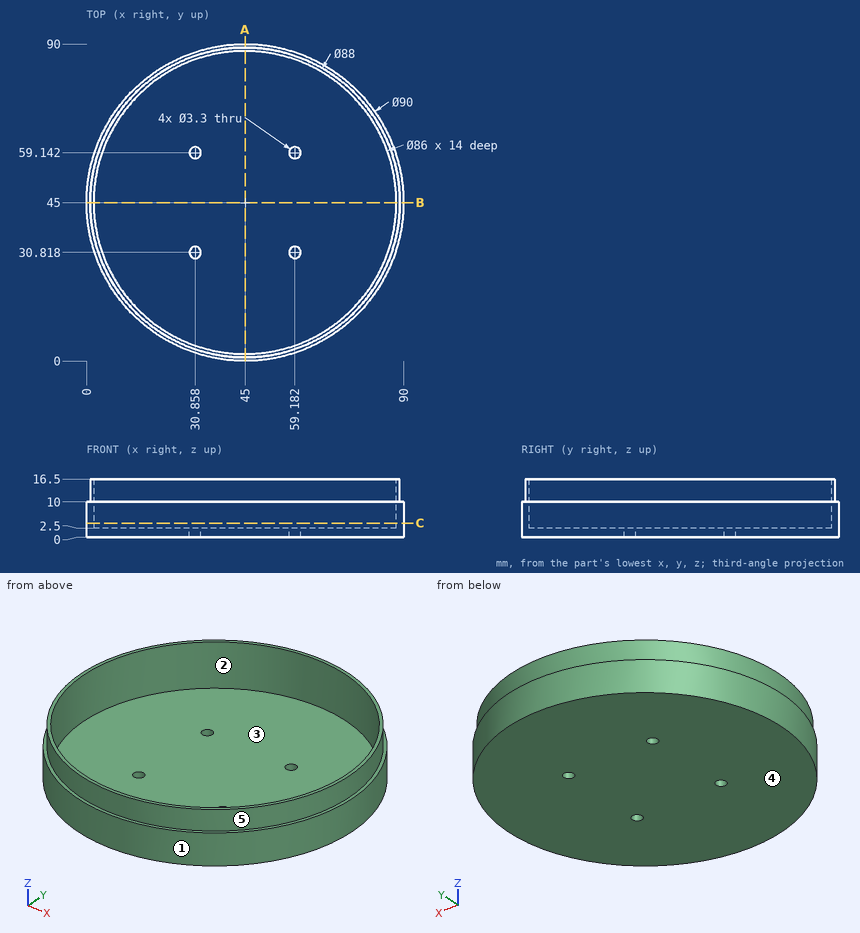
Check sheet for the drawn part. Datum: minimum x, y, z corner. Units: mm. A direction names the side the tool comes from. Give positions to 0.01 mm unless a question says otherwise; leave off trailing zeros. Write each loop counter-clockwise with the first axis right and the second up, starting at its lowest first coordinate (ties: lowest second). Pieces come first, ordered by that corner, then holes. Notation, with made-up numbers: (77.5, 35) - (114.5, 35) arc R26 cw to (114.5, 61) - close; hole circle Ø11 at (-6, 9). An arc over 180 degrees is marked (long way). Put each result on its own line as item: value.
1. Sectioned sample at C-C, the plane z = 4. Enter the section's corners in (x, y), plus the area to 3 significant figures.
Ans:
outline: circle Ø90 at (45, 45); hole circle Ø86 at (45, 45)
area: 553 mm²
2. Sectioned sample at A-A, the plane x = 45. Enter the section's corners in (y, z), plus the area to 3 significant figures.
Ans:
outline: (0, 0) - (90, 0) - (90, 10) - (89, 10) - (89, 16.5) - (88, 16.5) - (88, 2.5) - (2, 2.5) - (2, 16.5) - (1, 16.5) - (1, 10) - (0, 10) - close
area: 268 mm²
3. Draft check along Y on the marked faces 3, 4 and 5. Enter one of: +Y half, -Y half, draft (parallel to the pull), parting line (faces both ways), or undercut.
Ans:
face 3: undercut
face 4: draft
face 5: parting line
4. Go/stop test with flat-tipped pins: pin 1 (10 mm diameter, centred on x = 11, y = 58, fed in from +Z); pin 2 (3 mm diameter, centred on y = 66.5, z = 9.5, fed in from -X); pin 3 (3 mm diameter, centred on y = 17.5, z = 9.5, fed in from -X). Record where each tip stops, or that it passes through.
Ans:
pin 1: stops at z = 2.5
pin 2: stops at x = 4.69
pin 3: stops at x = 8.27
5. Thickness scan on line 1 (X direction, y = 60, z = 1.75); line 2 (Y direction, x = 45, z = 10.25); line 3 (Z direction, x = 38, y = 10.5). Record the ranges inside material, lowest first.
Ans:
line 1: x = 2.57 to 29.45, 32.27 to 57.77, 60.59 to 87.43
line 2: y = 1 to 2, 88 to 89
line 3: z = 0 to 2.5
6. Set-up check for the marked faces 1 and 2: record each of +Z, -Z, +X, -X, +Y, -Y from which the full face is reachable in a straight line by a thin tool's end or side.
Ans:
face 1: +Z, -Z
face 2: +Z
